Build history of the part. All positions in model axes, mm. Coordinates: 2 decimals unless noted, no trailing zeros. Order: outer loops, then holes, each group sorted by start corner. A loop starts at its lowest first (then second) coordinate and runs counter-clockwise, first axis right, second up. Notation, with made-up numbers: (37, 19.5) - (82, 19.5) arc R23 cw to (82, 37.5) - close; hole circle Ø3 at (-30.5, 18). An arc over 180 degrees is marked (long way). Answer as CSV lines item,"result". Start each with the question number.
Autodesk Inventor part; units mm, degrees
ref_plane "YZ Plane" through (0, 0, 0) normal (1, 0, 0) x (0, 1, 0)
ref_plane "XZ Plane" through (0, 0, 0) normal (0, 1, 0) x (-1, 0, 0)
ref_plane "XY Plane" through (0, 0, 0) normal (0, 0, 1) x (1, 0, 0)
sketch "Szkic1" plane through (0, 0, 0) normal (0, 1, 0) x (-1, 0, 0)
  circle A0 centre (0, 0) radius 12.5
  line L0 (-12.5, 12.5) -> (12.5, 12.5)
  line L1 (12.5, 12.5) -> (12.5, -12.5)
  line L2 (12.5, -12.5) -> (-12.5, -12.5)
  line L3 (-12.5, -12.5) -> (-12.5, 12.5)
  line L4 (-12.5, 12.5) -> (12.5, -12.5) construction
  line L5 (12.5, 12.5) -> (-12.5, -12.5) construction
  circle A1 centre (12.5, -12.5) radius 2.1
  circle A2 centre (-12.5, -12.5) radius 2.1
  circle A3 centre (-12.5, 12.5) radius 2.1
  circle A4 centre (12.5, 12.5) radius 2.1
  circle A5 centre (0, 0) radius 50.5
  line L6 (-25, 3.4426) -> (25, 3.4426)
  line L7 (25, 3.4426) -> (25, -3.4426)
  line L8 (25, -3.4426) -> (-25, -3.4426)
  line L9 (-25, -3.4426) -> (-25, 3.4426)
  line L10 (-25, 3.4426) -> (25, -3.4426) construction
  line L11 (25, 3.4426) -> (-25, -3.4426) construction
  circle A6 centre (-35.7881, 35.6295) radius 3
  line L12 (-35.7881, 38.6295) -> (-35.7881, 45.6295)
  line L13 (-35.7881, 32.6295) -> (-35.7881, 5.6295)
  line L14 (-35.7881, 5.6295) -> (-35.7881, 25.6295)
  line L15 (-45.7881, 45.6295) -> (-25.7881, 45.6295)
  line L16 (-25.7881, 45.6295) -> (-25.7881, 5.6295)
  line L17 (-25.7881, 5.6295) -> (-45.7881, 5.6295)
  line L18 (-45.7881, 5.6295) -> (-45.7881, 45.6295)
  line L19 (-45.7881, 45.6295) -> (-25.7881, 5.6295) construction
  line L20 (-25.7881, 45.6295) -> (-45.7881, 5.6295) construction
  line L21 (-40.7881, 49.6295) -> (-30.7881, 49.6295)
  line L22 (-30.7881, 49.6295) -> (-30.7881, 1.6295)
  line L23 (-30.7881, 1.6295) -> (-40.7881, 1.6295)
  line L24 (-40.7881, 1.6295) -> (-40.7881, 49.6295)
  line L25 (-40.7881, 49.6295) -> (-30.7881, 1.6295) construction
  line L26 (-30.7881, 49.6295) -> (-40.7881, 1.6295) construction
  circle A7 centre (-30.7881, 1.6295) radius 2.1
  circle A8 centre (-40.7881, 1.6295) radius 2.1
  circle A9 centre (-40.7881, 49.6295) radius 2.1
  circle A10 centre (-30.7881, 49.6295) radius 2.1
  line L27 (-46.2881, 46.1295) -> (-25.2881, 46.1295)
  line L28 (-25.2881, 46.1295) -> (-25.2881, 5.1295)
  line L29 (-25.2881, 5.1295) -> (-46.2881, 5.1295)
  line L30 (-46.2881, 5.1295) -> (-46.2881, 46.1295)
  line L31 (-46.2881, 46.1295) -> (-25.2881, 5.1295) construction
  line L32 (-25.2881, 46.1295) -> (-46.2881, 5.1295) construction
  line L33 (-35.7881, 45.6295) -> (-35.7881, 53.6295)
  line L34 (-35.7881, 53.6295) -> (-45.7881, 53.6295)
  line L35 (-45.7881, 53.6295) -> (-45.7881, 46.1295)
  line L36 (-35.7881, 53.6295) -> (-5.7881, 53.6295)
  line L37 (-18.25, 18.25) -> (18.25, 18.25)
  line L38 (18.25, 18.25) -> (18.25, -18.25)
  line L39 (18.25, -18.25) -> (-18.25, -18.25)
  line L40 (-18.25, -18.25) -> (-18.25, 18.25)
  line L41 (-18.25, 18.25) -> (18.25, -18.25) construction
  line L42 (18.25, 18.25) -> (-18.25, -18.25) construction
  line L43 (18.25, 18.25) -> (-5.7881, 53.6295)
  line L44 (-45.7881, 5.1295) -> (-45.7881, -2.8705)
  line L45 (-45.7881, -2.8705) -> (-18.25, -18.25)
  dimension "d9" = 101
  dimension "d0" = 25
  dimension "d1" = 25
  dimension "d2" = 25
  dimension "d3" = 4.2
  dimension "d4" = 4.2
  dimension "d5" = 4.2
  dimension "d6" = 4.2
  dimension "d13" = 50
  dimension "d17" = 6
  dimension "d18" = 7
  dimension "d19" = 27
  dimension "d20" = 20
  dimension "d21" = 20
  dimension "d22" = 40
  dimension "d23" = 10
  dimension "d24" = 48
  dimension "d25" = 4.2
  dimension "d26" = 4.2
  dimension "d27" = 4.2
  dimension "d28" = 4.2
  dimension "d29" = 21
  dimension "d30" = 41
  dimension "d31" = 8
  dimension "d32" = 10
  dimension "d33" = 30
  dimension "d34" = 36.5
  dimension "d35" = 36.5
  dimension "d36" = 8
extrude "Wyciągnięcie proste1" add sketch "Szkic1" along normal blind 3 contours L1 L8 A0 | A0 L6 L1 | L1 L6 L38 L8 | A0 L0 A4 L1 L6 | L8 L1 A1 L2 A0 | L1 A4 L0 A3 L3 L6 L40 L37 L38 | L8 L38 L39 L40 L3 A2 L2 A1 L1 | A0 L6 L3 A3 L0 | A0 L3 L6 | L2 A2 L3 L8 A0 | L8 L3 A0 | L3 L8 L40 L6 | L37 L40 L6 L9 L8 L45 L44 L29 L24 A8 L23 A7 L22 L28 A5 L43 | L40 L8 L9 L6 | A5 L28 L27 L22 A10 L21 L33 L36 L43 | L33 L21 A9 L24 L27 L35 L34 | L27 L33 L21 A10 L22 | L22 A7 L23 A8 L24 L29 | L33 L27 L24 A9 L21
fillet "Zaokrąglenie1" radius 0.5 2 edges at (25.2881, 1.5, 5.1295) (25.2881, 1.5, 46.1295)
fillet "Zaokrąglenie3" radius 3.5 3 edges at (45.7881, 1.5, 5.1295) (45.7881, 1.5, 46.1295) (45.7881, 1.5, 53.6295)
fillet "Zaokrąglenie4" radius 7 1 edges at (45.7881, 1.5, -2.8705)
fillet "Zaokrąglenie5" radius 70 1 edges at (18.25, 1.5, -18.25)
fillet "Zaokrąglenie6" radius 49 1 edges at (5.7881, 1.5, 53.6295)
fillet "Zaokrąglenie7" radius 49 1 edges at (-18.25, 1.5, 18.25)
fillet "Zaokrąglenie8" radius 7 1 edges at (-18.25, 1.5, -18.25)
properties part number "plyka zawor servo"
(1) Pull direction Z, two halves, no side cores. Call faces 1 (the cylindrical face through (44.79, 1.52, 47.18)), 2 (the cylindrical face through (17.9, 1.52, -15.93)), 3 (the flat face through (-9.294, 1.479, 31.431)): +Z half, -Z half, draft (parallel to the pull), parting line (faces both ways), or undercut.
(2) Band-saw the part on D-D on z = 15.5. List the corners of the cut face in (x, y).
(3) Drop flat-ended pins along their axis: pin 1 Ø1.5 at (y, z) = (1.5, 26.5) entering from -X; pin 2 Ø1 at (x, y) = (7, 1) entering from -Z; pin 3 Ø1 at (x, y) = (38.5, 2) entering from -Z. Give the stop position or say it passes through.
(4) Band-saw the part on C-C on x = 16.5. List the corners of the cut face in (y, z), plus the area to 3 significant figures.
(5) Probe L1, parallel to Z at x = 11, y = 2.75; L2, parallel to X at y = 1.3, z = -11; L3, parallel to Z at x = 30, y = 2.75. List the from-to ranges inside material, lowest first. Write a range as [from, to].
(6) Band-saw the part on A-A on y = 1.45. State how many separate pieces and enclosed holes the cut face has, plus the area to 3 significant figures.
(7) Band-saw the part on B-B on x = -1.5. List the corners of the cut face in (y, z), plus the area to 3 significant figures.
Filled in:
1,face 1,"undercut"
1,face 2,"-Z half"
1,face 3,"+Z half"
2,outline,"(-16.68, 0) - (25.29, 0) - (25.29, 3) - (-16.68, 3) - close"
3,pin 1,"stops at x = -12.74"
3,pin 2,"stops at z = -17.95"
3,pin 3,"stops at z = -7.22"
4,outline,"(0, -16.28) - (3, -16.28) - (3, 51.2) - (0, 51.2) - close"
4,area,"202 mm^2"
5,L1,"z = [-17.38, -13.97], [-11.03, -5.94], [5.94, 11.03], [13.97, 49.03]"
5,L2,"x = [-18.25, -13.97], [-11.03, -5.94], [5.94, 11.03], [13.97, 31.05]"
5,L3,"z = [-11.51, -0.32], [3.58, 5.13], [46.13, 47.68], [51.58, 53.6]"
6,separate pieces,"1"
6,enclosed holes,"9"
6,area,"2,350 mm^2"
7,outline,"(0, -18.25) - (3, -18.25) - (3, -12.41) - (0, -12.41) - close; (0, 12.41) - (3, 12.41) - (3, 40.63) - (0, 40.63) - close"
7,area,"102 mm^2"
